Input: part model. Units: mm. Frame: model coordinates. A direction names the side the tool comes from. Give positions to 0.01 mm unless a question says otherwise; leave off trailing zeros. Loops run counter-clockwise (first coordinate to the right, second up) from the corner with the lowest first, then second, coordinate; pieces in that order, holes last. Notation, with made-up numbers: (30.25, 86.25) -> (64.25, 86.25) arc R13 cw to (64.25, 106.25) -> close; hole circle Ø5 at (-15, 44). An arc over 180 degrees is marked (long way). Use CSV: the item, a comma, the result in double quotes.
```python
from build123d import *

# Parameters (mm, degrees)
F1_DEPTH = 300
F2_R     = 3.65
F3_DEPTH = 300


with BuildPart() as f1:
    # F0 (on Top) → F1 (new body)
    with BuildSketch(Plane.XY):
        with BuildLine():
            ThreePointArc((0, 2), (0.585786, 0.585786), (2, 0))
            Line((2, 0), (10.4, 0))
            Line((10.4, 0), (10.4, 0.5))
            Line((10.4, 0.5), (11, 0.5))
            Line((11, 0.5), (11, 1.7))
            Line((11, 1.7), (6.7, 1.7))
            Line((6.7, 1.7), (6.7, 3.7))
            Line((6.7, 3.7), (11.707107, 8.707107))
            ThreePointArc((11.707107, 8.707107), (12.03153, 8.92388), (12.414214, 9))
            ThreePointArc((12.414214, 9), (15.2, 8.447547), (17.985786, 9))
            ThreePointArc((17.985786, 9), (18.36847, 8.92388), (18.692893, 8.707107))
            Line((18.692893, 8.707107), (23.7, 3.7))
            Line((23.7, 3.7), (23.7, 1.7))
            Line((23.7, 1.7), (19.2, 1.7))
            Line((19.2, 1.7), (19.2, 0.5))
            Line((19.2, 0.5), (19.8, 0.5))
            Line((19.8, 0.5), (19.8, 0))
            Line((19.8, 0), (28, 0))
            ThreePointArc((28, 0), (29.414214, 0.585786), (30, 2))
            Line((30, 2), (30, 10.2))
            Line((30, 10.2), (29.5, 10.2))
            Line((29.5, 10.2), (29.5, 10.8))
            Line((29.5, 10.8), (28.3, 10.8))
            Line((28.3, 10.8), (28.3, 6.3))
            Line((28.3, 6.3), (26.3, 6.3))
            Line((26.3, 6.3), (21.292893, 11.307107))
            ThreePointArc((21.292893, 11.307107), (21.07612, 11.63153), (21, 12.014214))
            ThreePointArc((21, 12.014214), (21.552453, 14.8), (21, 17.585786))
            ThreePointArc((21, 17.585786), (21.07612, 17.96847), (21.292893, 18.292893))
            Line((21.292893, 18.292893), (26.3, 23.3))
            Line((26.3, 23.3), (28.3, 23.3))
            Line((28.3, 23.3), (28.3, 19))
            Line((28.3, 19), (29.5, 19))
            Line((29.5, 19), (29.5, 19.6))
            Line((29.5, 19.6), (30, 19.6))
            Line((30, 19.6), (30, 28))
            ThreePointArc((30, 28), (29.414214, 29.414214), (28, 30))
            Line((28, 30), (19.8, 30))
            Line((19.8, 30), (19.8, 29.5))
            Line((19.8, 29.5), (19.2, 29.5))
            Line((19.2, 29.5), (19.2, 28.3))
            Line((19.2, 28.3), (23.7, 28.3))
            Line((23.7, 28.3), (23.7, 26.3))
            Line((23.7, 26.3), (18.692893, 21.292893))
            ThreePointArc((18.692893, 21.292893), (18.36847, 21.07612), (17.985786, 21))
            ThreePointArc((17.985786, 21), (15.2, 21.552453), (12.414214, 21))
            ThreePointArc((12.414214, 21), (12.03153, 21.07612), (11.707107, 21.292893))
            Line((11.707107, 21.292893), (6.7, 26.3))
            Line((6.7, 26.3), (6.7, 28.3))
            Line((6.7, 28.3), (11, 28.3))
            Line((11, 28.3), (11, 29.5))
            Line((11, 29.5), (10.4, 29.5))
            Line((10.4, 29.5), (10.4, 30))
            Line((10.4, 30), (2, 30))
            ThreePointArc((2, 30), (0.585786, 29.414214), (0, 28))
            Line((0, 28), (0, 19.6))
            Line((0, 19.6), (0.5, 19.6))
            Line((0.5, 19.6), (0.5, 19))
            Line((0.5, 19), (1.7, 19))
            Line((1.7, 19), (1.7, 23.3))
            Line((1.7, 23.3), (3.7, 23.3))
            Line((3.7, 23.3), (8.707107, 18.292893))
            ThreePointArc((8.707107, 18.292893), (8.92388, 17.96847), (9, 17.585786))
            ThreePointArc((9, 17.585786), (8.447547, 14.8), (9, 12.014214))
            ThreePointArc((9, 12.014214), (8.92388, 11.63153), (8.707107, 11.307107))
            Line((8.707107, 11.307107), (3.7, 6.3))
            Line((3.7, 6.3), (1.7, 6.3))
            Line((1.7, 6.3), (1.7, 10.8))
            Line((1.7, 10.8), (0.5, 10.8))
            Line((0.5, 10.8), (0.5, 10.2))
            Line((0.5, 10.2), (0, 10.2))
            Line((0, 10.2), (0, 2))
        make_face()
    extrude(amount=F1_DEPTH)

    # F2 (on face) → F3 (cut)
    with BuildSketch(Plane.XY.offset(300)):
        with Locations((15, 15)):
            Circle(F2_R)
    extrude(amount=-F3_DEPTH, mode=Mode.SUBTRACT)


solid = f1.part
```
1) Mould query, pull axis X, two halves, no side actions, for faces 3 (the flat face through (0, 24, 148)), 4 (the cylindrical face through (11.354, 15.16, 152.1)), 5 (the cylindrical face through (15.24, 21.552, 147.9)), 6 (the flat face through (30, 6, 148)). Classes: pulls with the +X half, pulls with the -X half, needs draft (parallel to the pull), parting line crosses it, or undercut.
From the geometry:
face 3,"pulls with the -X half"
face 4,"undercut"
face 5,"undercut"
face 6,"pulls with the +X half"
2) Section query A-A (x = 15). Return loops of the section in (y, z), then the cut area to 3 significant figures.
From the geometry:
outline,"(8.45, 0) -> (11.35, 0) -> (11.35, 300) -> (8.45, 300) -> close; (18.65, 0) -> (21.55, 0) -> (21.55, 300) -> (18.65, 300) -> close"
area,"1,740 mm^2"
3) Reachability of faces 1 (the flat face through (11, 19, 0)), 2 (the flat face through (6, 21, 148)) from +Z, -Z, +X, -X, +Y, -Y: full face, straight path, thin tool, end or side. Return the list, or none.
From the geometry:
face 1,"-Z, +X, -X, +Y, -Y"
face 2,"+Z, -Z"
4) Ray query, line 1 (Y direction, x = 15, z = 221.5); line 2 (Y direction, x = 2.5, z = 166.5); line 3 (X direction, y = 20, z = 138). Return the intervals inside material, ascending.
From the geometry:
line 1,"y = 8.45 to 11.35, 18.65 to 21.55"
line 2,"y = 0 to 6.3, 23.3 to 30"
line 3,"x = 0 to 1.7, 7 to 23, 28.3 to 30"
5) Contact query for flat-ended pins moving along their axis: pin 1 (1.3 mm diameter, centred on x = 1, z = 175.5, fed in from +Y); pin 2 (0.5 mm diameter, centred on x = 19.5, z = 170.5, fed in from -Y). Output: stop coordinate, or through.
From the geometry:
pin 1,"stops at y = 29.97"
pin 2,"stops at y = 0.5"
